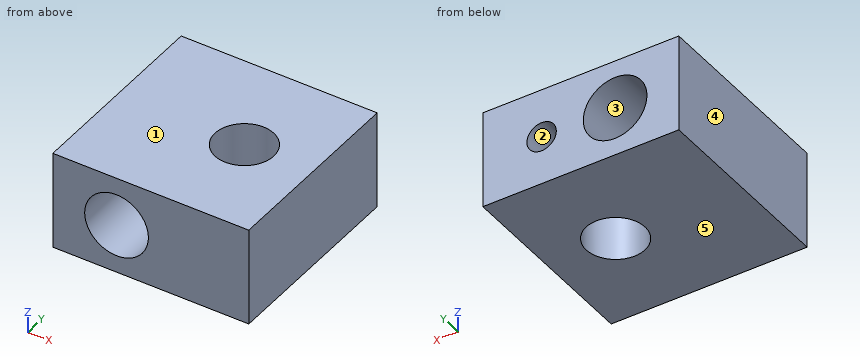
```python
from build123d import *

# Parameters (mm, degrees)
F0_W     = 20
F0_H     = 20
F0_R     = 3
F1_DEPTH = 10
F2_R     = 3.25
F3_DEPTH = 20.001
F2_R_2   = 1.5
F4_DEPTH = 5


with BuildPart() as f1:
    # F0 (on Top) → F1 (new body)
    with BuildSketch(Plane.XY):
        Rectangle(F0_W, F0_H)
        with Locations((3, 0)):
            Circle(F0_R, mode=Mode.SUBTRACT)
    extrude(amount=F1_DEPTH)

    # F2 (on face) → F3 (cut, through all)
    with BuildSketch(Plane(origin=(0, 10, 0), x_dir=(-1, 0, 0), z_dir=(0, 1, 0))):
        with Locations((3.5, 5)):
            Circle(F2_R)
    extrude(amount=-F3_DEPTH, mode=Mode.SUBTRACT)

    # F2 (on face) → F4 (cut)
    with BuildSketch(Plane(origin=(0, 10, 0), x_dir=(-1, 0, 0), z_dir=(0, 1, 0))):
        with Locations((-4, 5)):
            Circle(F2_R_2)
    extrude(amount=-F4_DEPTH, mode=Mode.SUBTRACT)


solid = f1.part
```
Model file for the job. Use its own axes, mm. Face numbers are marked on the shaded views. A direction names the side the tool comes from. Coordinates: 2 decimals unless noted, no trailing zeros. Loops run counter-clockwise (first coordinate to the right, second up) from the corner with the lowest first, then second, coordinate; pieces in that order, holes last. Notation, with made-up numbers: (34, 48) - (44, 48) arc R17 cw to (44, 78) - close; hole circle Ø1 at (-23.5, 26). An arc over 180 degrees is marked (long way). Answer as a JSON object with one key per item and string values. Group by question number.
(1) Two-plate mould, pull along X, no slides. Class the marked faces 3, 4 and 5: released by +X, released by -X, zero draft, split by the parting line, or undercut.
(2) Probe line 1 along Z through (x, y) = (4, 7.7); line 2 along Z through (x, y) = (-3.5, -1.75); line 3 along Y through (x, z) = (3, 6.75). List the from-to ranges inside material, lowest first.
(3) Cut at A-A (y = 0). Give the cut face in (x, z).
(4) Tool access for the marked faces 1 and 2: list every direction of +Z, -Z, +X, -X, +Y, -Y with a clear straight run to the whole face (end or side of a thin tool).
(5) Flat gauge pin, fed straight in: pin 1 (5 mm diameter, centred on x = 3, y = 0, fed in from -Z). Where does the tip first touch, or does it go through?
(6) Cut at B-B (z = 5). Give the cut face in (x, y).
(7) Cut at D-D (z = 1). Give the cut face in (x, y).
(8) Cut at C-C (x = -3.5). Give the cut face in (y, z).
Geometry says:
{
 "1": {"face 3": "undercut", "face 4": "released by -X", "face 5": "zero draft"},
 "2": {"line 1": "z = 0 to 3.5, 6.5 to 10", "line 2": "z = 0 to 1.75, 8.25 to 10", "line 3": "y = -10 to -3, 3 to 10"},
 "3": {"outline": "(-10, 0) - (0, 0) - (0, 10) - (-10, 10) - close; (6, 0) - (10, 0) - (10, 10) - (6, 10) - close; hole circle Ø6.5 at (-3.5, 5)"},
 "4": {"face 1": "+Z, +X, -X, +Y, -Y", "face 2": "+Y"},
 "5": {"pin 1": "passes through"},
 "6": {"outline": "(-10, -10) - (-6.75, -10) - (-6.75, 10) - (-10, 10) - close; (-0.25, -10) - (10, -10) - (10, 10) - (5.5, 10) - (5.5, 5) - (2.5, 5) - (2.5, 10) - (-0.25, 10) - close; hole circle Ø6 at (3, 0)"},
 "7": {"outline": "(-10, -10) - (10, -10) - (10, 10) - (-10, 10) - close; hole circle Ø6 at (3, 0)"},
 "8": {"outline": "(-10, 0) - (10, 0) - (10, 1.75) - (-10, 1.75) - close; (-10, 8.25) - (10, 8.25) - (10, 10) - (-10, 10) - close"}
}
